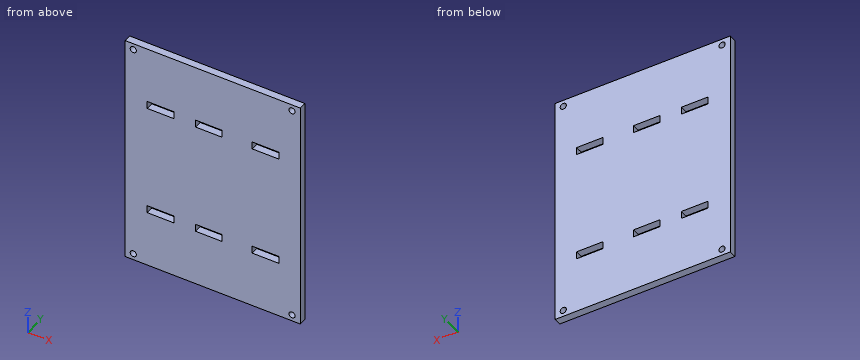
from build123d import *

# Parameters (mm, degrees)
SKETCH1_W           = 125.999999968
SKETCH1_H           = 165.999999978
BOSS_EXTRUDE1_DEPTH = 5.334
SKETCH9_W           = 19.270046927
SKETCH9_H           = 5.334
SKETCH9_W_2         = 18.946166646
SKETCH9_W_3         = 19.104051368
CUT_EXTRUDE1_DEPTH  = 164.220324554
SKETCH10_R          = 2.223521257
SKETCH10_R_2        = 2.222212396
SKETCH10_R_3        = 2.223409271
SKETCH10_R_4        = 2.239695252
CUT_EXTRUDE2_DEPTH  = 164.220324554


with BuildPart() as part:
    # Sketch1 → Boss-Extrude1 (new body)
    with BuildSketch(Plane(origin=(0, 0, 0), x_dir=(1, 0, 0), z_dir=(0, 1, 0))):
        with Locations((38.977787599, 44.330097126)):
            Rectangle(SKETCH1_W, SKETCH1_H)
    extrude(amount=BOSS_EXTRUDE1_DEPTH)

    # Sketch9 → Cut-Extrude1 (cut, through all)
    with BuildSketch(Plane(origin=(0, 5.334, 0), x_dir=(1, 0, 0), z_dir=(0, 1, 0))):
        with Locations((1.575384394, 4.262022439)):
            Rectangle(SKETCH9_W, SKETCH9_H)
        with Locations((1.575384394, 84.398171813)):
            Rectangle(SKETCH9_W, SKETCH9_H)
        with Locations((36.148083105, 84.398171813)):
            Rectangle(SKETCH9_W_2, SKETCH9_H)
        with Locations((76.961283755, 84.398171813)):
            Rectangle(SKETCH9_W_3, SKETCH9_H)
        with Locations((76.961283755, 4.262022439)):
            Rectangle(SKETCH9_W_3, SKETCH9_H)
        with Locations((36.148083105, 4.262022439)):
            Rectangle(SKETCH9_W_2, SKETCH9_H)
    extrude(amount=-CUT_EXTRUDE1_DEPTH, mode=Mode.SUBTRACT)

    # Sketch10 → Cut-Extrude2 (cut, through all)
    with BuildSketch(Plane(origin=(0, 5.334, 0), x_dir=(1, 0, 0), z_dir=(0, 1, 0))):
        with Locations(Location((96.035287599, -34.119902874, 0), (0, 0, 270))):
            Circle(SKETCH10_R)
        with Locations(Location((96.035287599, 122.780097126, 0), (0, 0, 270))):
            Circle(SKETCH10_R_2)
        with Locations(Location((-18.079712401, 122.780097126, 0), (0, 0, 270))):
            Circle(SKETCH10_R_3)
        with Locations(Location((-18.079712401, -34.119902874, 0), (0, 0, 270))):
            Circle(SKETCH10_R_4)
    extrude(amount=-CUT_EXTRUDE2_DEPTH, mode=Mode.SUBTRACT)


solid = part.part
Source: CAD feature listing. Evaluate the final solid. Frame: model axes, mm. Coordinates: 2 decimals unless noted, no trailing zeros. Loops run counter-clockwise (first coordinate to the right, second up) from the corner with the lowest first, then second, coordinate; pieces in that order, holes last. Notation, with made-up numbers: (89.25, 22) - (129.25, 22) arc R21 cw to (129.25, 42) - close; hole circle Ø6 at (49, 88). An arc over 180 degrees is marked (long way). Return JSON: item names as keys, results as strings.
Q1. Section A-A, the plane x = 36. Return loops of the section in (y, z).
Results:
{"outline": "(0, -127.33) - (5.33, -127.33) - (5.33, -87.07) - (0, -87.07) - close; (0, -81.73) - (5.33, -81.73) - (5.33, -6.93) - (0, -6.93) - close; (0, -1.6) - (5.33, -1.6) - (5.33, 38.67) - (0, 38.67) - close"}
Q2. Section B-B, the plane z = -85. Return loops of the section in (x, y) (3 decimals).
Results:
{"outline": "(-24.022, 0) - (-8.06, 0) - (-8.06, 5.334) - (-24.022, 5.334) - close; (11.21, 0) - (26.675, 0) - (26.675, 5.334) - (11.21, 5.334) - close; (45.621, 0) - (67.409, 0) - (67.409, 5.334) - (45.621, 5.334) - close; (86.513, 0) - (101.978, 0) - (101.978, 5.334) - (86.513, 5.334) - close"}
Q3. Section C-C, the plane y = 3.5. Give the number of separate pieces and of enclosed holes in the cut face, plus the area to 3 significant figures.
Results:
{"separate pieces": "1", "enclosed holes": "10", "area": "20,200 mm2"}
Q4. Material intervals for line 1 along Z through (x, y) = (33.5, 2.4); line 2 along X through (y, z) = (3.15, -6) (3 decimals), sorted ascending.
Results:
{"line 1": "-127.33 to -87.07, -81.73 to -6.93, -1.6 to 38.67", "line 2": "-24.022 to -8.06, 11.21 to 26.675, 45.621 to 67.409, 86.513 to 101.978"}
